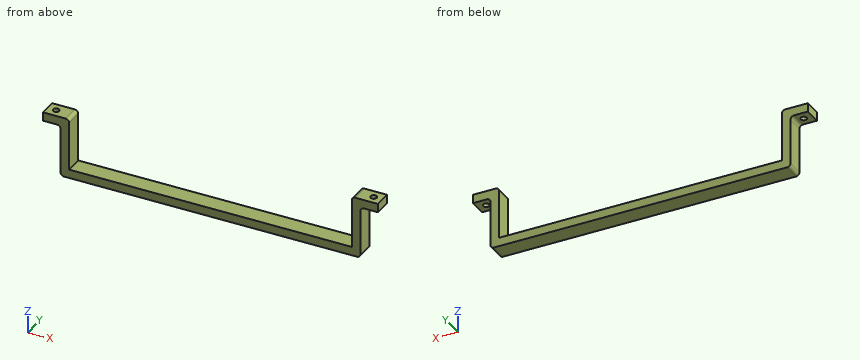
from build123d import *

# Parameters (mm, degrees)
F0_W     = 10
F0_H     = 5
F0_W_2   = 81
F1_DEPTH = 10
F2_R     = 1.75
F3_DEPTH = 35.001
F4_R     = 2


with BuildPart() as f1:
    # F0 (on Front) → F1 (new body)
    with BuildSketch(Plane.XZ):
        with Locations((-91, 32.5)):
            Rectangle(F0_W, F0_H)
        Polygon((-86, 0), (-81, 0), (-81, 5), (-81, 35), (-86, 35), (-86, 30), align=None)
        with Locations((-40.5, 2.5)):
            Rectangle(F0_W_2, F0_H)
    extrude(amount=F1_DEPTH)

    # F2 (on face) → F3 (cut, through all)
    with BuildSketch(Plane.XY.offset(35)):
        with Locations((-91, -5)):
            Circle(F2_R)
    extrude(amount=-F3_DEPTH, mode=Mode.SUBTRACT)

    # F4
    f4_edges = [f1.edges().sort_by_distance(p)[0] for p in [
        (-81, -5, 35),
        (-86, -5, 30),
        (-86, -5, 0),
    ]]
    fillet(f4_edges, radius=F4_R)

    # F5: F1 across plane


with BuildPart() as f1_1:
    add(f1.part)
    add(f1.part.mirror(Plane.YZ))


solid = f1_1.part
CAD build for the part. Positions are in the model's coordinates, mm. Give positions to 0.01 mm unless a question says otherwise; leave off trailing zeros. Write each loop counter-clockwise with the first axis right and the second up, starting at its lowest first coordinate (ties: lowest second). Pieces come first, ordered by that corner, then holes. Notation, with made-up numbers: (8, -10) - (64, -10) arc R11 ccw to (64, 8) - close; hole circle Ø1 at (77.25, 33.5). An arc over 180 degrees is marked (long way). Put each result on its own line as item: value.
(1) Saw through at B-B (z = 15). List the corners of the cut face in (x, y), then the cut area to 3 significant figures.
Working result:
outline: (-86, -10) - (-81, -10) - (-81, 0) - (-86, 0) - close; (81, -10) - (86, -10) - (86, 0) - (81, 0) - close
area: 100 mm^2
(2) Drop flat-ended pins along their axis: pin 1 Ø1 at (y, z) = (-7, 12) entering from +X; pin 2 Ø5 at (y, z) = (-3.5, 21.5) entering from -X; pin 3 Ø2 at (x, y) = (22, -3.5) entering from +Z. Give the stop position or say it passes through.
Working result:
pin 1: x = 86
pin 2: x = -86
pin 3: z = 5
(3) Wall check: L1, parallel to X at y = -0.25, z = 15.5; L2, parallel to Y at x = 91, z = 31.9; L3, parallel to X at y = -8.5, z = 32. Give the ranges that are in metal, low to high.
Working result:
L1: -86 to -81, 81 to 86
L2: -10 to -6.75, -3.25 to 0
L3: -96 to -81, 81 to 96
(4) Saw through at C-C (x = -91). List the corners of the cut face in (y, z), then the cut area to 3 significant figures.
Working result:
outline: (-10, 30) - (-6.75, 30) - (-6.75, 35) - (-10, 35) - close; (-3.25, 30) - (0, 30) - (0, 35) - (-3.25, 35) - close
area: 32.5 mm^2
(5) Saw through at A-A (y = -5). List the corners of the cut face in (x, z), then the cut area to 3 significant figures.
Working result:
outline: (-96, 30) - (-92.75, 30) - (-92.75, 35) - (-96, 35) - close; (-89.25, 30) - (-88, 30) arc R2 cw to (-86, 28) - (-86, 2) arc R2 ccw to (-84, 0) - (84, 0) arc R2 ccw to (86, 2) - (86, 28) arc R2 cw to (88, 30) - (89.25, 30) - (89.25, 35) - (83, 35) arc R2 ccw to (81, 33) - (81, 5) - (-81, 5) - (-81, 33) arc R2 ccw to (-83, 35) - (-89.25, 35) - close; (92.75, 30) - (96, 30) - (96, 35) - (92.75, 35) - close
area: 1,220 mm^2
(6) Saw through at D-D (x = -71). List the corners of the cut face in (y, z).
Working result:
outline: (-10, 0) - (0, 0) - (0, 5) - (-10, 5) - close
